Check sheet for the modelled part. Datum: model origin and axes. Units: mm. Face numbers are marked on the shaded views. A direction names the side the tool comes from. Give positions to 0.01 mm unless a question says otherwise; leave off trailing zeros. Write each loop counter-clockwise with the first axis right and the second up, starting at its lowest first coordinate (ties: lowest second). Pieces come first, ordered by that corner, then holes. Notation, with made-up numbers: (-9.5, 87.5) -> (33.5, 87.5) arc R23 ccw to (33.5, 103.5) -> close; hole circle Ø9 at (-13.75, -32.5). An arc over 180 degrees is marked (long way). Return JSON: item names as keys, results as strings.
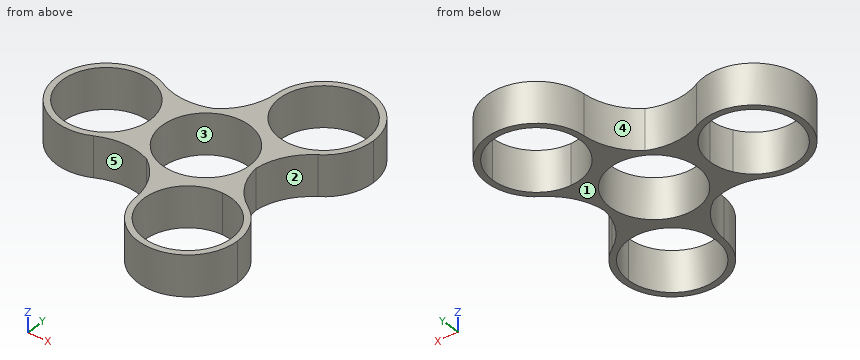
from build123d import *

# Parameters (mm, degrees)
F0_R        = 11
F1_DEPTH    = 10.16
F2_T1_DEPTH = 10.16


# Not quite as in the source:
# - a fillet or chamfer that OpenCascade refuses, or shapes differently, is made with other operations: its cross-section is extruded or revolved along the edge and cut away or added


with BuildPart() as f1:
    # F0 (on Top) → F1 (new body)
    with BuildSketch(Plane.XY):
        with BuildLine():
            ThreePointArc((-6.2500001721, -10.8253174479), (-12.5, 3.1e-08), (-6.2500001185, 10.8253174789))
            Line((-6.2500001185, 10.8253174789), (-14.177453734, 6.2484))
            ThreePointArc((-14.177453734, 6.2484), (-12.929018134, 3.2344098428), (-12.5032, 0))
            ThreePointArc((-12.5032, 0), (-12.929018134, -3.2344098428), (-14.177453734, -6.2484))
            Line((-14.177453734, -6.2484), (-6.2500001721, -10.8253174479))
        make_face()
        with BuildLine():
            Line((-15.4737205584, 5.5), (-14.177453734, 6.2484))
            ThreePointArc((-14.177453734, 6.2484), (-37.4968, 0), (-14.177453734, -6.2484))
            Line((-14.177453734, -6.2484), (-15.4737205584, -5.5))
            ThreePointArc((-15.4737205584, -5.5), (-36, 0), (-15.4737205584, 5.5))
        make_face()
        with BuildLine():
            Line((12.5, -9.1538350946), (12.5, 0))
            ThreePointArc((12.5, 0), (6.2499999139, -10.825317597), (-6.2500001721, -10.8253174479))
            Line((-6.2500001721, -10.8253174479), (1.677453734, -15.4022350946))
            ThreePointArc((1.677453734, -15.4022350946), (6.2516, -10.8280888286), (12.5, -9.1538350946))
        make_face()
        with BuildLine():
            ThreePointArc((24.9968, -21.6506350946), (21.3365720231, -12.8140630715), (12.5, -9.1538350946))
            Line((12.5, -9.1538350946), (12.5, -10.6506350946))
            ThreePointArc((12.5, -10.6506350946), (20.2781745931, -13.8724605016), (23.5, -21.6506350946))
            ThreePointArc((23.5, -21.6506350946), (9.6529905039, -32.2758191838), (2.9737205584, -16.1506350946))
            Line((2.9737205584, -16.1506350946), (1.677453734, -15.4022350946))
            ThreePointArc((1.677453734, -15.4022350946), (9.2655901572, -33.7216169606), (24.9968, -21.6506350946))
        make_face()
        with BuildLine():
            Line((12.5, -10.6506350946), (12.5, -9.1538350946))
            ThreePointArc((12.5, -9.1538350946), (6.2516, -10.8280888286), (1.677453734, -15.4022350946))
            Line((1.677453734, -15.4022350946), (2.9737205584, -16.1506350946))
            ThreePointArc((2.9737205584, -16.1506350946), (7, -12.124355653), (12.5, -10.6506350946))
        make_face()
        with BuildLine():
            ThreePointArc((-6.2500001721, -10.8253174479), (6.2499999139, -10.825317597), (12.5, 0))
            ThreePointArc((12.5, 0), (6.2499999408, 10.8253175815), (-6.2500001185, 10.8253174789))
            ThreePointArc((-6.2500001185, 10.8253174789), (-12.5, 3.1e-08), (-6.2500001721, -10.8253174479))
        make_face()
        Circle(F0_R, mode=Mode.SUBTRACT)
        with BuildLine():
            ThreePointArc((-6.2500001185, 10.8253174789), (6.2499999408, 10.8253175815), (12.5, 0))
            Line((12.5, 0), (12.5, 9.1538350946))
            ThreePointArc((12.5, 9.1538350946), (6.2516, 10.8280888286), (1.677453734, 15.4022350946))
            Line((1.677453734, 15.4022350946), (-6.2500001185, 10.8253174789))
        make_face()
        with BuildLine():
            ThreePointArc((1.677453734, 15.4022350946), (6.2516, 10.8280888286), (12.5, 9.1538350946))
            Line((12.5, 9.1538350946), (12.5, 10.6506350946))
            ThreePointArc((12.5, 10.6506350946), (7, 12.124355653), (2.9737205584, 16.1506350946))
            Line((2.9737205584, 16.1506350946), (1.677453734, 15.4022350946))
        make_face()
        with BuildLine():
            Line((12.5, 10.6506350946), (12.5, 9.1538350946))
            ThreePointArc((12.5, 9.1538350946), (21.3365720231, 12.8140630715), (24.9968, 21.6506350946))
            ThreePointArc((24.9968, 21.6506350946), (9.2655901572, 33.7216169606), (1.677453734, 15.4022350946))
            Line((1.677453734, 15.4022350946), (2.9737205584, 16.1506350946))
            ThreePointArc((2.9737205584, 16.1506350946), (9.6529905039, 32.2758191838), (23.5, 21.6506350946))
            ThreePointArc((23.5, 21.6506350946), (20.2781745931, 13.8724605016), (12.5, 10.6506350946))
        make_face()
        with BuildLine():
            ThreePointArc((-12.5032, 0), (-12.929018134, 3.2344098428), (-14.177453734, 6.2484))
            Line((-14.177453734, 6.2484), (-15.4737205584, 5.5))
            ThreePointArc((-15.4737205584, 5.5), (-14.3748159108, 2.8470094961), (-14, 0))
            ThreePointArc((-14, 0), (-14.3748159108, -2.8470094961), (-15.4737205584, -5.5))
            Line((-15.4737205584, -5.5), (-14.177453734, -6.2484))
            ThreePointArc((-14.177453734, -6.2484), (-12.929018134, -3.2344098428), (-12.5032, 0))
        make_face()
    extrude(amount=F1_DEPTH)

    # F2: fillet of radius 15.24 on 6 edges, made by hand

    # F2_s2 → F2_t1 (join)
    with BuildSketch(Plane.XY):
        with BuildLine():
            ThreePointArc((-4.9300135605, -11.5874120735), (-12.1072951031, -9.5520710185), (-19.3906654504, -11.1671561353))
            ThreePointArc((-19.3906654504, -11.1671561353), (-16.42385767, -9.0895430565), (-14.177453734, -6.2484))
            Line((-14.177453734, -6.2484), (-4.9300135605, -11.5874120735))
        make_face()
        with BuildLine():
            ThreePointArc((12.5, -1.5241890523), (14.3259837123, 5.7091896211), (19.3663736264, 11.2092308086))
            ThreePointArc((19.3663736264, 11.2092308086), (16.0837040307, 9.6787064421), (12.5, 9.1538350946))
            Line((12.5, 9.1538350946), (12.5, -1.5241890523))
        make_face()
        with BuildLine():
            ThreePointArc((19.3663736264, -11.2092308086), (14.3259837123, -5.7091896211), (12.5, 1.5241890523))
            Line((12.5, 1.5241890523), (12.5, -9.1538350946))
            ThreePointArc((12.5, -9.1538350946), (16.0837040307, -9.6787064421), (19.3663736264, -11.2092308086))
        make_face()
        with BuildLine():
            ThreePointArc((0.024291824, 22.3763869439), (-2.2186886092, 15.2612606396), (-7.5699864395, 10.0632230212))
            Line((-7.5699864395, 10.0632230212), (1.677453734, 15.4022350946))
            ThreePointArc((1.677453734, 15.4022350946), (0.3401536393, 18.7682494986), (0.024291824, 22.3763869439))
        make_face()
        with BuildLine():
            ThreePointArc((-4.9300135605, 11.5874120735), (-12.1072951031, 9.5520710185), (-19.3906654504, 11.1671561353))
            ThreePointArc((-19.3906654504, 11.1671561353), (-16.42385767, 9.0895430565), (-14.177453734, 6.2484))
            Line((-14.177453734, 6.2484), (-4.9300135605, 11.5874120735))
        make_face()
        with BuildLine():
            ThreePointArc((-7.5699864395, -10.0632230212), (-2.2186886092, -15.2612606396), (0.024291824, -22.3763869439))
            ThreePointArc((0.024291824, -22.3763869439), (0.3401536393, -18.7682494986), (1.677453734, -15.4022350946))
            Line((1.677453734, -15.4022350946), (-7.5699864395, -10.0632230212))
        make_face()
    extrude(amount=F2_T1_DEPTH)


solid = f1.part
(1) Cross-section at A-A on x = -25. Enter the section's corners in (y, z).
Reply:
{"outline": "(-12.5, 0) -> (-11, 0) -> (-11, 10.16) -> (-12.5, 10.16) -> close; (11, 0) -> (12.5, 0) -> (12.5, 10.16) -> (11, 10.16) -> close"}
(2) Thickness scan on L1, parallel to Y at x = 12.5, z = 7.25; L2, parallel to Y at x = -25, z = 2.5; L3, parallel to Y at x = 22, z = 9.5. Record the ranges inside material, lowest first.
Reply:
{"L1": "-34.15 to -32.65, -10.65 to 10.65, 32.65 to 34.15", "L2": "-12.5 to -11, 11 to 12.5", "L3": "-29.77 to -27.2, -16.11 to -13.53, 13.53 to 16.11, 27.2 to 29.77"}
(3) Cross-section at B-B on z = 8.75. Enter the section's corners in (x, y).
Reply:
{"outline": "(-19.39, -11.17) arc R15.24 cw to (-6.29, -10.89) arc R15.24 cw to (0.02, -22.38) arc R12.5 ccw (long way) to (19.37, -11.21) arc R15.24 cw to (12.58, 0) arc R15.24 cw to (19.37, 11.21) arc R12.5 ccw (long way) to (0.02, 22.38) arc R15.24 cw to (-6.29, 10.89) arc R15.24 cw to (-19.39, 11.17) arc R12.5 ccw (long way) to start; hole circle Ø22 at (-25, 0); hole circle Ø22 at (0, 0); hole circle Ø22 at (12.5, -21.65); hole circle Ø22 at (12.5, 21.65)"}
(4) Release check for a two-part mould opening along X. For the marked faces 1, 2 and 3 record: pulls with the +X half, pulls with the -X half, needs draft (parallel to the pull), parting line crosses it, or undercut.
Reply:
{"face 1": "needs draft", "face 2": "pulls with the +X half", "face 3": "undercut"}
(5) Cross-section at C-C on y = -18.5. Enter the section's corners in (x, z).
Reply:
{"outline": "(-0.71, 0) -> (1.96, 0) -> (1.96, 10.16) -> (-0.71, 10.16) -> close; (23.04, 0) -> (24.59, 0) -> (24.59, 10.16) -> (23.04, 10.16) -> close"}
(6) Set-up check for the marked faces 4 and 5: record each of +Z, -Z, +X, -X, +Y, -Y from which the full face is reachable in a straight line by a thin tool's end or side.
Reply:
{"face 4": "+Z, -Z, +Y", "face 5": "+Z, -Z, -Y"}
(7) Cross-section at D-D on y = -1. Enter the section's corners in (x, z).
Reply:
{"outline": "(-37.46, 0) -> (-35.95, 0) -> (-35.95, 10.16) -> (-37.46, 10.16) -> close; (-14.05, 0) -> (-10.95, 0) -> (-10.95, 10.16) -> (-14.05, 10.16) -> close; (10.95, 0) -> (12.71, 0) -> (12.71, 10.16) -> (10.95, 10.16) -> close"}
(8) Depth check by flat-ended pin: pin 1 Ø20 at (x, y) = (-25, 0) entering from -Z; pin 2 Ø4 at (x, z) = (-28.5, 2) entering from +Y; pin 3 Ø1 at (y, z) = (12, 2) entering from +X. Enter the tip coordinate at first touch or a pass-through.
Reply:
{"pin 1": "through", "pin 2": "y = 12.41", "pin 3": "x = 21.01"}
